CAD build for the part. Positions are in the model's coordinates, mm. A direction names the side the tool comes from. Coordinates: 2 decimals unless noted, no trailing zeros. Loops run counter-clockwise (first coordinate to the right, second up) from the corner with the lowest first, then second, coordinate; pieces in that order, holes last. Notation, with made-up numbers: (79.5, 89.5) -> (101.5, 89.5) arc R6 cw to (101.5, 99.5) -> close; hole circle Ø3 at (-26, 45). An arc over 180 degrees is marked (long way). Write item = value, one per line. Start each with the question number.
(1) Flat gauge pins, fed straight in: P1, Ø10, axis at x = 18, y = 17.5, coming from the -Z side; P2, Ø1.7, axis at y = -5.5, z = 1.5, coming from the +X side; P3, Ø5, axis at x = 12, z = -15, coming from the +Y side. Where does each tip first touch, or does it go through?
(2) Band-saw the part on A-A (y = 14). Write the cut outline in (x, z).
(3) Band-saw the part on B-B (z = 1). Write the cut outline in (x, y), and give its area (3 significant figures).
(4) Tool access for faces 1 (the face through (1, 11, 7.377)), 2 (the face through (8, 11, 6.16)), 3 (the face through (5, 0, -9)): list every direction of +Z, -Z, +X, -X, +Y, -Y with a clear straight run to the whole face (end or side of a thin tool).
(5) Pull direction Z, two halves, no side cores. Call faces 4 (the face through (1, 0, -7)), 5 (the face through (8, 0, -7)): +Z half, -Z half, draft (parallel to the pull), parting line (faces both ways), or undercut.
(6) Band-saw the part on D-D (y = -7). Write the cut outline in (x, z).
(7) Drill centre lines: line 1 (X direction, y = 12.5, z = -10); line 2 (Z direction, x = -3, y = -21); line 3 (Z direction, x = 2, y = -12). Where is each one in solid material? Low to high. Write a range as from..to.
(8) Band-saw the part on C-C (x = 5.5). Write the cut outline in (y, z), and give its area (3 significant figures).
```python
from build123d import *

# Parameters (mm, degrees)
F2_W      = 1.825324
F2_H      = 15.819468
F3_DEPTH  = 50.8
F4_W      = 2.966151
F4_H      = 21.295437
F5_DEPTH  = 50.8
F6_W      = 1.630356
F6_H      = 20.682175
F7_DEPTH  = 50.8
F8_W      = 1.825323
F8_H      = 19.774335
F9_DEPTH  = 50.8
F10_W     = 17.340573
F10_H     = 2.129544
F11_DEPTH = 50.8
F12_W     = 19.470113
F12_H     = 3.422481
F13_DEPTH = 50.8
F14_W     = 20.078553
F14_H     = 2.433764
F15_DEPTH = 50.8
F16_W     = 25.250305
F16_H     = 1.521244
F17_DEPTH = 50.8


with BuildPart() as f1:
    # F0 (on Front) → F1 (revolve)
    with BuildSketch(Plane.XZ):
        with BuildLine():
            Line((-24.29125, 0), (24.29125, 0))
            ThreePointArc((24.29125, 0), (0, 24.29125), (-24.29125, 0))
        make_face()
    revolve(axis=Axis((0, 0, 0), (1, 0, 0)))

    # F2 (on Front) → F3 (cut)
    with BuildSketch(Plane.XZ):
        with Locations((-7.073127, -3.878812)):
            Rectangle(F2_W, F2_H)
    extrude(amount=-F3_DEPTH, mode=Mode.SUBTRACT)

    # F4 (on Front) → F5 (cut)
    with BuildSketch(Plane.XZ):
        with Locations((1.483075, -3.270371)):
            Rectangle(F4_W, F4_H)
    extrude(amount=-F5_DEPTH, mode=Mode.SUBTRACT)

    # F6 (on Front) → F7 (cut)
    with BuildSketch(Plane.XZ):
        with Locations((-3.491047, -3.679285)):
            Rectangle(F6_W, F6_H)
    extrude(amount=-F7_DEPTH, mode=Mode.SUBTRACT)

    # F8 (on Front) → F9 (cut)
    with BuildSketch(Plane.XZ):
        with Locations((8.44212, -3.726701)):
            Rectangle(F8_W, F8_H)
    extrude(amount=-F9_DEPTH, mode=Mode.SUBTRACT)

    # F10 (on Front) → F11 (cut)
    with BuildSketch(Plane.XZ):
        with Locations((1.140828, 7.833679)):
            Rectangle(F10_W, F10_H)
    extrude(amount=F11_DEPTH, mode=Mode.SUBTRACT)

    # F12 (on Front) → F13 (cut)
    with BuildSketch(Plane.XZ):
        with Locations((0.684495, 1.71124)):
            Rectangle(F12_W, F12_H)
    extrude(amount=F13_DEPTH, mode=Mode.SUBTRACT)

    # F14 (on Front) → F15 (cut)
    with BuildSketch(Plane.XZ):
        with Locations((0.684496, -4.487253)):
            Rectangle(F14_W, F14_H)
    extrude(amount=F15_DEPTH, mode=Mode.SUBTRACT)

    # F16 (on Front) → F17 (cut)
    with BuildSketch(Plane.XZ):
        with Locations((4.183032, -9.41451)):
            Rectangle(F16_W, F16_H)
    extrude(amount=F17_DEPTH, mode=Mode.SUBTRACT)


solid = f1.part
```
Findings below:
q1.P1 = -13.63
q1.P2 = 23.8
q1.P3 = 17.63
q2.outline = circle Ø39.7 at (0, 0); hole (-7.99, -11.79) -> (-6.16, -11.79) -> (-6.16, 4.03) -> (-7.99, 4.03) -> close; hole (-4.31, -14.02) -> (-2.68, -14.02) -> (-2.68, 6.66) -> (-4.31, 6.66) -> close; hole (0, -13.92) -> (2.97, -13.92) -> (2.97, 7.38) -> (0, 7.38) -> close; hole (7.53, -13.61) -> (9.35, -13.61) -> (9.35, 6.16) -> (7.53, 6.16) -> close
q3.outline = (-9.05, -22.52) -> (-9.05, 0) -> (-7.99, 0) -> (-7.99, 22.92) arc R24.27 ccw to start; (-6.16, 0) -> (-4.31, 0) -> (-4.31, 23.89) arc R24.27 ccw to (-6.16, 23.48) -> close; (-2.68, 0) -> (0, 0) -> (0, 24.27) arc R24.27 ccw to (-2.68, 24.12) -> close; (2.97, 0) -> (7.53, 0) -> (7.53, 23.07) arc R24.27 ccw to (2.97, 24.09) -> close; (9.35, 0) -> (10.42, 0) -> (10.42, -21.92) arc R24.27 ccw to (9.35, 22.4) -> close
q3.area = 1,200 mm²
q4.face_1 = +Y, -Y
q4.face_2 = +Y
q4.face_3 = -Y
q5.face_4 = undercut
q5.face_5 = undercut
q6.outline = circle Ø46.52 at (0, 0); hole (-9.35, -5.7) -> (10.72, -5.7) -> (10.72, -3.27) -> (-9.35, -3.27) -> close; hole (-9.05, 0) -> (10.42, 0) -> (10.42, 3.42) -> (-9.05, 3.42) -> close; hole (-8.44, -10.18) -> (16.81, -10.18) -> (16.81, -8.65) -> (-8.44, -8.65) -> close; hole (-7.53, 6.77) -> (9.81, 6.77) -> (9.81, 8.9) -> (-7.53, 8.9) -> close
q7.line_1 = -18.27..-7.99, -6.16..-4.31, -2.68..0, 2.97..7.53, 9.35..18.27
q7.line_2 = -11.83..-10.18, -8.65..-5.7, -3.27..0, 3.42..6.77, 8.9..11.83
q7.line_3 = -21.03..-10.18, -8.65..-5.7, -3.27..0, 3.42..6.77, 8.9..21.03
q8.outline = (-23.66, 0) arc R23.66 ccw to (-23.43, -3.27) -> (0, -3.27) -> (0, -5.7) -> (-22.96, -5.7) arc R23.66 ccw to (-22.02, -8.65) -> (0, -8.65) -> (0, -10.18) -> (-21.36, -10.18) arc R23.66 ccw (long way) to (-21.92, 8.9) -> (0, 8.9) -> (0, 6.77) -> (-22.67, 6.77) arc R23.66 ccw to (-23.41, 3.42) -> (0, 3.42) -> (0, 0) -> close
q8.area = 1,540 mm²
